Autodesk Inventor part; units mm, degrees
ref_plane "YZ Plane" through (0, 0, 0) normal (1, 0, 0) x (0, 1, 0)
ref_plane "XZ Plane" through (0, 0, 0) normal (0, 1, 0) x (-1, 0, 0)
ref_plane "XY Plane" through (0, 0, 0) normal (0, 0, 1) x (1, 0, 0)
sketch "Sketch1" plane through (0, 0, 0) normal (0, 1, 0) x (-1, 0, 0)
  circle A0 centre (0, 0) radius 10
  dimension "d0" = 20
extrude "Extrusion1" add sketch "Sketch1" along normal blind 10
sketch "Sketch2" plane through (0, 0, 0) normal (1, 0, 0) x (0, 1, 0)
  line L0 (10, -10) -> (10, 10)
  line L1 (10, 0) -> (10, 12)
  line L2 (10, 0) -> (10, -12)
  circle A0 centre (10, -10) radius 12.15
  circle A1 centre (10, 10) radius 12.15
  circle A2 centre (16.9009, 0) radius 12.15
  line L3 (30.6793, 0) -> (0, 0)
  point P0 (29.0509, 0)
  point P1 (4.7509, 0)
  dimension "d5" = 24.3
  dimension "d6" = 24.3
  dimension "d3" = 12
  dimension "d4" = 12
  dimension "d7" = 24.3
revolve "Revolution1" add sketch "Sketch2" angle 360 about axis through (0, 30.6793, 0) along (0, -1, 0) picked at (16.7279, 5.8245) picked at (22.9675, 2.0985) contours L3 A2 A0 L0 | L0 A0 L3 | A0 L0 A2 A1 | A1 A2 L3 | A0 A2 L0
sketch "Sketch3" plane through (0, 0, 0) normal (0, -1, 0) x (1, 0, 0)
  circle A0 centre (0, 0) radius 20
  dimension "d9" = 40
extrude "Extrusion2" add sketch "Sketch3" along normal blind 5
chamfer "Chamfer1" distance 5 angle 45 1 edges at (10, 0, 0)
properties part number "Foot Swivel"
Could you check a few things on this model? Use its own coordinates, in mm. Coordinates: 2 decimals unless noted, no trailing zeros. Loops run counter-clockwise (first coordinate to the right, second up) from the corner with the lowest first, then second, coordinate; pieces in that order, holes last.
1. Imagine slicing it at D-D (y = 8). Please give me the cut outline in (x, z), and give its area (3 significant figures).
2. Imagine slicing it at B-B (z = 0). Please give me the cut outline in (x, y), and give its area (3 significant figures).
3. I need wall thicknesses on L1, parallel to Y at x = 16.5, z = -10; L2, parallel to Y at x = 10, z = 2; L3, parallel to Y at x = -3.5, z = -2.5. Which ranges of each line are inside material? Lowest first, please.
4. Imagine slicing it at A-A (x = 0). Please give me the cut outline in (y, z), and give its area (3 significant figures).
5. Imagine slicing it at C-C (y = 2.5). Please give me the cut outline in (x, z).
6. For P1, Ø1, axis at x = 4, z = -1, coming from the +Y side; P2, Ø12, axis at x = -1.5, z = 8.5, coming from the +Y side; P3, Ø12, axis at x = -6, y = 0, coming from the -Z side, each with a flat end and sliding along its axis, tell me the tip position at first contact or that it passes through.
7. We'd pull the mould along Y, two halves only. Please class faces 1 (the face through (2.236, 4.687, 10.068)), 2 (the face through (2.17, 7.46, 9.76)), 3 (the face through (0, -5, 0)), 4 (the face through (3, 0, 15)): released by +Y, released by -Y, zero draft, split by the parting line, or undercut.
Computed values:
1. outline: circle Ø20 at (0, 0)
1. area: 314 mm2
2. outline: (-20, -5) - (20, -5) - (20, 0) - (15, 0) - (10, 5) - (10, 10) arc R12.15 ccw (long way) to (-10, 10) - (-10, 5) - (-15, 0) - (-20, 0) - close
2. area: 815 mm2
3. L1: y = -5 to 0
3. L2: y = -5 to 4.8, 10.3 to 23.51
3. L3: y = -5 to 28.26
4. outline: (-5, -20) - (0, -20) - (0, -15) - (5, -10) - (10, -10) arc R12.15 ccw (long way) to (10, 10) - (5, 10) - (0, 15) - (0, 20) - (-5, 20) - close
4. area: 815 mm2
5. outline: circle Ø25 at (0, 0)
6. P1: stops at y = 28.5
6. P2: stops at y = 28.76
6. P3: stops at z = -20
7. face 1: undercut
7. face 2: undercut
7. face 3: released by -Y
7. face 4: released by +Y
